from build123d import *

# Parameters (mm, degrees)
BOSS_EXTRUDE3_DEPTH     = 7.5
CUT_EXTRUDE4_DEPTH      = 1.5
BOSS_EXTRUDE5_DEPTH     = 1.5
SHAFT_HOLE_REACH        = 34.838
SHAFT_HOLE_END_RADIUS   = 175
SKETCH7_R               = 1.5
CUT_EXTRUDE6_DEPTH      = 178.777126726
CUT_EXTRUDE6_DEPTH_BACK = 178.777126726
SKETCH8_R               = 1.5


with BuildPart() as part:
    # Sketch1 → Boss-Extrude3 (new, symmetric)
    with BuildSketch(Plane.XY):
        with BuildLine():
            Line((-157.569240482, 27.783708427), (-172.341356777, 30.388431092))
            ThreePointArc((-172.341356777, 30.388431092), (-175, 0), (-172.341356777, -30.388431092))
            Line((-172.341356777, -30.388431092), (-157.569240482, -27.783708427))
            ThreePointArc((-157.569240482, -27.783708427), (-160, 0), (-157.569240482, 27.783708427))
        make_face()
    extrude(amount=BOSS_EXTRUDE3_DEPTH, both=True)

    # Sketch1_6 → Cut-Extrude4 (cut, symmetric)
    with BuildSketch(Plane.XY):
        with BuildLine():
            Line((-157.569240482, 27.783708427), (-172.341356777, 30.388431092))
            ThreePointArc((-172.341356777, 30.388431092), (-175, 0), (-172.341356777, -30.388431092))
            Line((-172.341356777, -30.388431092), (-157.569240482, -27.783708427))
            ThreePointArc((-157.569240482, -27.783708427), (-160, 0), (-157.569240482, 27.783708427))
        make_face()
    extrude(amount=CUT_EXTRUDE4_DEPTH, both=True, mode=Mode.SUBTRACT)


with BuildPart() as cut_extrude4_piece_1:
    # of the separate pieces the step leaves, piece 1, a body of its own (cut_extrude4_pieces)
    add(part.part.solids().sort_by_distance((-172.341356777, 30.388431092, -1.5))[0])



with BuildPart() as cut_extrude4_piece_2:
    # of the separate pieces the step leaves, piece 2, a body of its own (cut_extrude4_pieces)
    add(part.part.solids().sort_by_distance((-172.341356777, 30.388431092, 7.5))[0])


with BuildPart() as cut_extrude4_piece_1_1:
    add(cut_extrude4_piece_1.part)

    add(cut_extrude4_piece_2.part)  # Boss-Extrude5 merges Cut-Extrude4 piece 2
    # Sketch6 → Boss-Extrude5 (add, symmetric)
    with BuildSketch(Plane.XY):
        with BuildLine():
            Line((-159.824122084, 7.5), (-174.839211849, 7.5))
            ThreePointArc((-174.839211849, 7.5), (-175, 0), (-174.839211849, -7.5))
            Line((-174.839211849, -7.5), (-159.824122084, -7.5))
            ThreePointArc((-159.824122084, -7.5), (-160, 0), (-159.824122084, 7.5))
        make_face()
    extrude(amount=BOSS_EXTRUDE5_DEPTH, both=True)

    # shaft hole: up to this cylinder (the profile starts inside it)
    shaft_hole_end = Plane(origin=(0, 0, 0), z_dir=(0, 0, -1)) * Cylinder(SHAFT_HOLE_END_RADIUS, 420.676, mode=Mode.PRIVATE)
    # Sketch7 → shaft hole (cut, up to the surface)
    with BuildSketch(Plane(origin=(-167.5, 0, 0), x_dir=(0, 0, -1), z_dir=(1, 0, 0)), mode=Mode.PRIVATE) as shaft_hole_sk1:
        Circle(SKETCH7_R)
    shaft_hole_tool1 = extrude(shaft_hole_sk1.sketch, amount=-SHAFT_HOLE_REACH, mode=Mode.PRIVATE) & shaft_hole_end
    add(shaft_hole_tool1.solids().sort_by_distance((-167.5, 0, 0))[0], mode=Mode.SUBTRACT)

    # Sketch8 → Cut-Extrude6 (cut, two sides: drawn at the far end of the back side and taken through both)
    with BuildSketch(Plane.XY.offset(-CUT_EXTRUDE6_DEPTH_BACK)):
        with Locations((-166.306502189, 19.95989303)):
            Circle(SKETCH8_R)
        with Locations((-167.201226072, 10)):
            Circle(SKETCH8_R)
        with Locations((-167.201226072, -10)):
            Circle(SKETCH8_R)
        with Locations((-166.306502189, -19.95989303)):
            Circle(SKETCH8_R)
    extrude(amount=CUT_EXTRUDE6_DEPTH + CUT_EXTRUDE6_DEPTH_BACK, mode=Mode.SUBTRACT)


solid = cut_extrude4_piece_1_1.part
Model file for the job. Use its own axes, mm. A direction names the side the tool comes from. Give positions to 0.01 mm unless a question says otherwise; leave off trailing zeros. Order: outer loops, then holes, each group sorted by start corner. A loop starts at its lowest first (then second) coordinate and runs counter-clockwise, first axis right, second up. Notation, with made-up numbers: (84.5, 83.5) - (108.5, 83.5) arc R25 cw to (108.5, 98.5) - close; hole circle Ø10 at (-27.75, 80). An arc over 180 degrees is marked (long way). Write item = value, one per line. Start each with the question number.
1. Cut at A-A, the plane y = 22. List the corners of the cut face in (x, z), and give its area (3 significant figures).
2. Cut at C-C, the plane x = -169.5. List the corners of the cut face in (y, z), and give its area (3 significant figures).
3. Two-plate mould, pull along Z, no slides. Class faces 1 (the cylindrical face through (-167.805, -19.894, -4.542)), 2 (the flat face through (-167, 7.5, 0)), 3 (the flat face through (-168, -19, -1.5)), 4 (the flat face through (-166, 0, -7.5)): pulls with the +Z half, pulls with the -Z half, needs draft (parallel to the pull), parting line crosses it, or undercut.
4. Probe line 1 along Z through (x, y) = (-167.25, 13.5); line 2 along Y through (x, z) = (-165, 5). List the from-to ranges inside material, lowest first.
5. Cut at D-D, the plane y = 10. List the corners of the cut face in (x, z).
6. Cut at B-B, the plane z = 4.5. List the corners of the cut face in (x, y), and give its area (3 significant figures).
7. Drop flat-ended pins along their axis: P1, Ø4, axis at x = -169, z = 0, coming from the +Y side; P2, Ø3.5, axis at x = -165, z = -0.5, coming from the -Y side; P3, Ø8, axis at x = -162.5, z = 2, coming from the -Y side. Give the stop position or say it passes through.
8. Which spindle directions (+Z, -Z, +X, -X, +Y, -Y) get a long thin tool onto all of the face, cutting with end or side? Do faces 5 (the flat face through (-168, 19, 1.5)), 6 (the cylindrical face through (-167.805, -19.894, 4.458)), 7 (the flat face through (-167.5, 0, 0)), 8 (the flat face through (-168, -19, 1.5)). Say none if no direction does.
Taken from the geometry:
q1.outline = (-173.61, -7.5) - (-158.48, -7.5) - (-158.48, -1.5) - (-173.61, -1.5) - close; (-173.61, 1.5) - (-158.48, 1.5) - (-158.48, 7.5) - (-173.61, 7.5) - close
q1.area = 182 mm²
q2.outline = (-29.89, -7.5) - (29.89, -7.5) - (29.89, -1.5) - (7.5, -1.5) - (7.5, 1.5) - (29.89, 1.5) - (29.89, 7.5) - (-29.89, 7.5) - (-29.89, 1.5) - (-7.5, 1.5) - (-7.5, -1.5) - (-29.89, -1.5) - close; hole circle Ø3 at (0, 0)
q2.area = 755 mm²
q3.face_1 = needs draft
q3.face_2 = undercut
q3.face_3 = undercut
q3.face_4 = pulls with the -Z half
q4.line_1 = -7.5 to -1.5, 1.5 to 7.5
q4.line_2 = -29.09 to -20.7, -19.22 to 19.22, 20.7 to 29.09
q5.outline = (-174.71, -7.5) - (-168.7, -7.5) - (-168.7, -1.5) - (-174.71, -1.5) - close; (-174.71, 1.5) - (-168.7, 1.5) - (-168.7, 7.5) - (-174.71, 7.5) - close; (-165.7, -7.5) - (-159.69, -7.5) - (-159.69, -1.5) - (-165.7, -1.5) - close; (-165.7, 1.5) - (-159.69, 1.5) - (-159.69, 7.5) - (-165.7, 7.5) - close
q6.outline = (-172.34, -30.39) - (-157.57, -27.78) arc R160 cw to (-157.57, 27.78) - (-172.34, 30.39) arc R175 ccw to start; hole circle Ø3 at (-167.2, -10); hole circle Ø3 at (-167.2, 10); hole circle Ø3 at (-166.31, -19.96); hole circle Ø3 at (-166.31, 19.96)
q6.area = 849 mm²
q7.P1 = 30.03
q7.P2 = -29.35
q7.P3 = -29.36
q8.face_5 = +X, -X, +Y
q8.face_6 = +Z, -Z
q8.face_7 = -X
q8.face_8 = +X, -X, -Y
